Input: dimensioned drawing with shaded views. Units: mm. Origin: part minimum x, y, z. Give positions to 0.01 mm unless a question says otherwise; leave off trailing zeros. Write each loop counter-clockwise with the first axis right and the second up, starting at its lowest first coordinate (ties: lowest second). Pieces come first, ordered by that corner, then holes. Notation, with made-up numbers: (49, -24.75) -> (79, -24.75) arc R24 cw to (79, -4.75) -> close; hole circle Ø3 at (29, 43). An arc over 180 degrees is marked (long way). Answer as a JSON object with one key per item and string values. Group by question number.
(1) Section query D-D on y = 22.25. Output: boundary loops of the cut face in (x, z) (1 decimal).
(2) Section query A-A on y = 16. Output: boundary loops of the cut face in (x, z).
(3) Material intervals for probe 1 along Y at (x, z) = (16, 1.65); probe 2 along X at (y, z) = (22.5, 2.5); probe 3 along X at (y, z) = (22, 3.7), sorted ascending.
(4) Contact query for flat-ended pins moving along their axis: pin 1 Ø3 at (x, y) = (26.83, 9.75) entering from +Z; pin 2 Ø1.5 at (y, z) = (26, 4.5) entering from +X (1 decimal); pin 3 Ø1.5 at (x, z) = (10, 3) entering from +Y. Output: stop coordinate, or through.
(5) Draft query along X for the marked faces 1, 2 and 3. Return one class per face: +X half, -X half, draft (parallel to the pull), parting line (faces both ways), or undercut.
(6) Section query C-C on x = 20. Output: boundary loops of the cut face in (y, z).
(7) Section query B-B on z = 1.3. State how many separate pieces and enclosed holes the cut face has, plus the area to 3 significant figures.
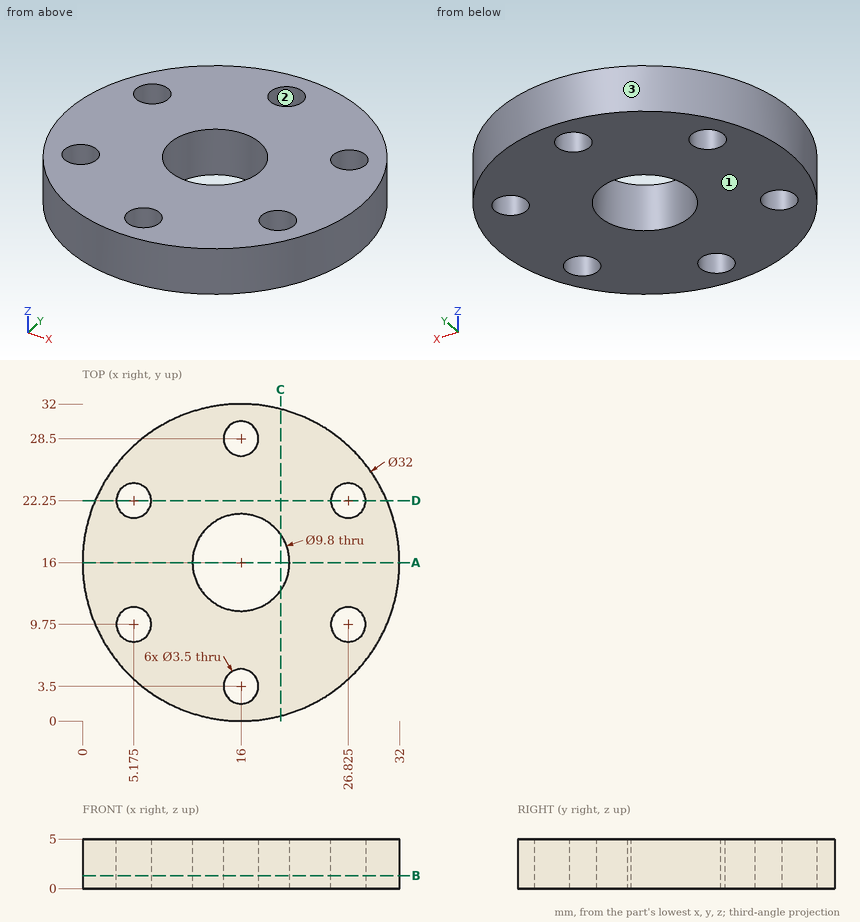
Answer list:
{
 "1": {"outline": "(1.3, 0) -> (3.4, 0) -> (3.4, 5) -> (1.3, 5) -> close; (6.9, 0) -> (25.1, 0) -> (25.1, 5) -> (6.9, 5) -> close; (28.6, 0) -> (30.7, 0) -> (30.7, 5) -> (28.6, 5) -> close"},
 "2": {"outline": "(0, 0) -> (11.1, 0) -> (11.1, 5) -> (0, 5) -> close; (20.9, 0) -> (32, 0) -> (32, 5) -> (20.9, 5) -> close"},
 "3": {"probe 1": "0 to 1.75, 5.25 to 11.1, 20.9 to 26.75, 30.25 to 32", "probe 2": "1.38 to 3.44, 6.91 to 25.09, 28.56 to 30.62", "probe 3": "1.17 to 3.44, 6.91 to 25.09, 28.56 to 30.83"},
 "4": {"pin 1": "through", "pin 2": "x = 29.1", "pin 3": "y = 31.11"},
 "5": {"face 1": "draft", "face 2": "undercut", "face 3": "parting line"},
 "6": {"outline": "(0.51, 0) -> (13.17, 0) -> (13.17, 5) -> (0.51, 5) -> close; (18.83, 0) -> (31.49, 0) -> (31.49, 5) -> (18.83, 5) -> close"},
 "7": {"separate pieces": "1", "enclosed holes": "7", "area": "671 mm2"}
}
